Autodesk Inventor part; units mm, degrees
ref_plane "YZ Plane" through (0, 0, 0) normal (1, 0, 0) x (0, 1, 0)
ref_plane "XZ Plane" through (0, 0, 0) normal (0, 1, 0) x (-1, 0, 0)
ref_plane "XY Plane" through (0, 0, 0) normal (0, 0, 1) x (1, 0, 0)
sketch "Sketch1" plane through (0, 0, 0) normal (0, 1, 0) x (-1, 0, 0)
  line L0 (-55.88, 45.72) -> (55.88, 45.72)
  line L1 (55.88, 45.72) -> (55.88, -45.72)
  line L2 (55.88, -45.72) -> (-55.88, -45.72)
  line L3 (-55.88, -45.72) -> (-55.88, 45.72)
  line L4 (-55.88, 45.72) -> (55.88, -45.72) construction
  line L5 (55.88, 45.72) -> (-55.88, -45.72) construction
  circle A0 centre (10.16, 0) radius 45.72
  point P0 (0, 0)
  point P1 (10.16, -45.72)
  point P2 (10.16, 45.72)
  dimension "d0" = 111.76
  dimension "d1" = 91.44
extrude "Extrusion1" add sketch "Sketch1" along normal blind 22.098 contours L0 A0 L2 L3 | A0
sketch "Sketch2" plane through (55.88, 0, -45.72) normal (0, 0, -1) x (-1, 0, 0)
  line L0 (66.04, 22.098) -> (0, 22.098)
  line L1 (66.04, 0) -> (0, 0)
  line L2 (0, 22.098) -> (10.16, 22.098)
  line L3 (10.16, 22.098) -> (10.16, 0)
  line L4 (10.16, 0) -> (0, 0)
  line L5 (0, 0) -> (0, 22.098)
  line L6 (5.08, 22.098) -> (5.08, 0)
  line L7 (0, 11.049) -> (10.16, 11.049)
  line L8 (0, 20.574) -> (10.16, 20.574)
  line L9 (10.16, 20.574) -> (10.16, 1.524)
  line L10 (10.16, 1.524) -> (0, 1.524)
  line L11 (0, 1.524) -> (0, 20.574)
  line L12 (0, 20.574) -> (10.16, 1.524) construction
  line L13 (10.16, 20.574) -> (0, 1.524) construction
  line L14 (10.16, 22.098) -> (22.225, 22.098)
  line L15 (22.225, 22.098) -> (22.225, 0)
  line L16 (22.225, 0) -> (10.16, 0)
  line L17 (10.16, 0) -> (10.16, 22.098)
  line L18 (10.16, 20.574) -> (22.225, 22.098)
  line L19 (22.225, 0) -> (10.16, 1.524)
  line L20 (5.08, 1.524) -> (10.16, 1.524)
  line L21 (5.08, 20.574) -> (10.16, 20.574)
  point P0 (55.88, 0)
  point P1 (5.08, 11.049)
  dimension "d4" = 10.16
  dimension "d5" = 19.05
  dimension "d6" = 12.065
extrude "Extrusion2" cut sketch "Sketch2" against normal blind 254 contours L18 L3 L0 | L3 L8 L6 L0 | L1 L3 L19 | L6 L8 L5 L0 | L1 L6 L10 L3 | L1 L5 L10 L6
sketch "Sketch3" plane through (0, 22.098, 0) normal (0, 1, 0) x (1, 0, 0)
  line L0 (-10.16, -45.72) -> (33.655, -45.72)
  line L1 (33.655, -45.72) -> (33.655, -23.368)
  line L2 (33.655, 45.72) -> (33.655, -45.72)
  line L3 (33.655, -23.368) -> (-49.457, -23.368)
  arc A0 (-10.16, 45.72) -> (-10.16, -45.72) centre (-10.16, 0) ccw
  line L4 (45.72, 45.72) -> (33.655, 45.72)
  line L5 (33.655, 45.72) -> (33.655, 28.448)
  line L6 (33.655, 28.448) -> (-45.9515, 28.448)
  line L7 (55.88, -45.72) -> (55.88, 45.72)
  line L8 (55.88, 28.448) -> (16.637, 28.448)
  line L9 (16.637, 28.448) -> (16.637, -23.368)
  circle A1 centre (-9.271, 2.54) radius 25.908
  point P0 (0, 0)
  dimension "d9" = 22.352
  dimension "d10" = 17.272
  dimension "d11" = 39.243
extrude "Extrusion3" cut sketch "Sketch3" against normal blind 254 contours A1
properties part number "fan"
Geometry check sheet. Reference: the model listing, model coordinates, mm. A direction names the side the tool comes from. Coordinates: 2 decimals unless noted, no trailing zeros. Order: outer loops, then holes, each group sorted by start corner. A loop starts at its lowest first (then second) coordinate and runs counter-clockwise, first axis right, second up. Notation, with made-up numbers: (-28, 69) - (-14, 69) arc R18 cw to (-14, 85) - close; hole circle Ø4 at (-38, 36.5). An arc over 180 degrees is marked (long way). Answer in a Markdown table with one row per item. Add a question column.
1) Cross-section at C-C, the plane z = 0. Record the cut outline in (x, y) (3 decimals).
2) Release check for a two-part mould opening along Z. For faces 3 (the flat face through (51, 20.574, -1)), 4 (the cylindrical face through (-14.89, 11.2, 22.75)), 5 (the flat face through (23, 11, 45.72)) record: +Z half, -Z half, draft (parallel to the pull), parting line (faces both ways), or undercut.
3) Cross-section at A-A, the plane y = 18. Record the cut outline in (x, z), then the cut area to 3 significant figures.
4) Cross-section at B-B, the plane x = -15.5. Record the cut outline in (y, z).
5) Cross-section at D-D, the plane z = 27.5. Record the cut outline in (x, y) (3 decimals).
6) Material ranges on line 1 along Z through (x, y) = (-29.5, 15.5); line 2 along Z through (x, y) = (13, 13.5); line 3 along X through (y, z) = (4, -24.5), recorded low to high. Write a range as [from, to].
7) Gauge pin test, flat ends, axial feed: P1, Ø3, axis at x = 53, z = 12.5, coming from the +Y side; P2, Ø11, axis at x = 48.5, z = 4, coming from the -Y side; P3, Ø6, axis at x = 13.5, z = -1, coming from the +Y side; P4, Ø2, axis at x = 40.5, z = -30, coming from the +Y side. Record the tip position at first contact, or that the pin passes through.
8) Set-up check for faces 1 (the flat face through (51, 1.524, -1)), 2 (the flat face through (9, 0, 21)): record each of +Z, -Z, +X, -X, +Y, -Y from which the full face is reachable in a straight line by a thin tool's end or side.
Check result:
| question | item | result |
|---|---|---|
| 1 | outline | (-55.88, 0) - (-35.054, 0) - (-35.054, 22.098) - (-55.88, 22.098) - close; (16.512, 0) - (33.655, 0) - (45.72, 1.524) - (55.88, 1.524) - (55.88, 20.574) - (45.72, 20.574) - (33.655, 22.098) - (16.512, 22.098) - close |
| 2 | face 3 | draft |
| 2 | face 4 | undercut |
| 2 | face 5 | +Z half |
| 3 | outline | (-10.16, -45.72) - (55.88, -45.72) - (55.88, 45.72) - (-10.16, 45.72) arc R45.72 ccw to start; hole circle Ø51.82 at (-9.27, -2.54) |
| 3 | area | 7,210 mm² |
| 4 | outline | (0, -45.41) - (22.1, -45.41) - (22.1, -27.69) - (0, -27.69) - close; (0, 22.61) - (22.1, 22.61) - (22.1, 45.41) - (0, 45.41) - close |
| 5 | outline | (-46.685, 0) - (33.655, 0) - (45.72, 1.524) - (55.88, 1.524) - (55.88, 20.574) - (45.72, 20.574) - (33.655, 22.098) - (-46.685, 22.098) - close |
| 6 | line 1 | z = [-41.43, -18.73], [13.65, 41.43] |
| 6 | line 2 | z = [-45.72, -15.78], [10.7, 45.72] |
| 6 | line 3 | x = [-48.76, -23.02], [4.48, 55.88] |
| 7 | P1 | stops at y = 20.57 |
| 7 | P2 | stops at y = 1.18 |
| 7 | P3 | passes through |
| 7 | P4 | stops at y = 21.36 |
| 8 | face 1 | +Z, -Z, +X, -Y |
| 8 | face 2 | +Z, -Z, +X, -X, -Y |
